from build123d import *

# Parameters (mm, degrees)
SKETCH_W    = 200
SKETCH_H    = 45
PAD_DEPTH   = 19
FILLET_R    = 5
THICKNESS_T = -1


with BuildPart() as part:
    # Sketch → Pad (new body)
    with BuildSketch(Plane.XY):
        Rectangle(SKETCH_W, SKETCH_H)
    extrude(amount=PAD_DEPTH)

    # Fillet
    fillet_edges = [part.edges().sort_by_distance(p)[0] for p in [
        (-100, -22.5, 9.5),
        (-100, 22.5, 9.5),
        (100, -22.5, 9.5),
        (100, 22.5, 9.5),
    ]]
    fillet(fillet_edges, radius=FILLET_R)

    # Thickness
    thickness_openings = [part.faces().sort_by_distance(p)[0] for p in [
        (0, 0, 19),
    ]]
    offset(amount=THICKNESS_T, openings=thickness_openings)


solid = part.part
Can you work these out from the model? Positions are in its coordinate system, mm. A direction names the side the tool comes from. Give positions to 0.01 mm unless a question says otherwise; leave off trailing zeros. Loops run counter-clockwise (first coordinate to the right, second up) from the corner with the lowest first, then second, coordinate; pieces in that order, holes last. Notation, with made-up numbers: (5, -9) - (10, -9) arc R20 ccw to (10, 6) - close; hole circle Ø4 at (84, 89). An arc over 180 degrees is marked (long way). One line per item, written item: value.
(1) On a 3-axis mill with a long thin cutter (end or side, diameter ignored), from which of +Z, -Z, +X, -X, +Y, -Y can I reach the whole of each face in a straight line? I mean faces 4 (the face through (-1, 0, 0)), 5 (the face through (-99, 0, 10)). Say none if no direction works.
Verdict:
face 4: -Z, +X, -X, +Y, -Y
face 5: +Z
(2) I'm going to push a flat-ended pin straight in: pin 1 (10 mm diameter, centred on x = -66.5, y = -7, fed in from +Z). Where does the tip first touch, or does it pass through?
Verdict:
pin 1: z = 1
(3) If we section it at C-C, the plane x = 44: List the corners of the cut face in (y, z) for me, plus the area to 3 significant figures.
Verdict:
outline: (-22.5, 0) - (22.5, 0) - (22.5, 19) - (21.5, 19) - (21.5, 1) - (-21.5, 1) - (-21.5, 19) - (-22.5, 19) - close
area: 81.0 mm^2
(4) If we mould it in two halves opening along X, with no side actions, what happens to faces 1 (the face through (-1, 21.5, 10)), 2 (the face through (-98.57, 21, 9.63)), 3 (the face through (-1, 22.5, 9))? For each: released by +X, released by -X, zero draft, split by the parting line, or undercut.
Verdict:
face 1: undercut
face 2: released by -X
face 3: zero draft
(5) If we section it at A-A, the plane y = -2.5: List the corners of the cut face in (x, z) for me, plus the area to 3 significant figures.
Verdict:
outline: (-100, 0) - (100, 0) - (100, 19) - (99, 19) - (99, 1) - (-99, 1) - (-99, 19) - (-100, 19) - close
area: 236 mm^2
(6) I need wall thicknesses on line 1 along X through (y, z) = (4, 3.75); line 2 along Y through (x, z) = (67.5, 9.25); line 3 along Z through (x, y) = (-66, 16). Which ranges of each line are inside material? Lowest first, please.
Verdict:
line 1: -100 to -99, 99 to 100
line 2: -22.5 to -21.5, 21.5 to 22.5
line 3: 0 to 1
(7) If we section it at B-B, the plane z = 15: List the corners of the cut face in (x, y) for me.
Verdict:
outline: (-100, -17.5) arc R5 ccw to (-95, -22.5) - (95, -22.5) arc R5 ccw to (100, -17.5) - (100, 17.5) arc R5 ccw to (95, 22.5) - (-95, 22.5) arc R5 ccw to (-100, 17.5) - close; hole (-99, -17.5) arc R4 ccw to (-95, -21.5) - (95, -21.5) arc R4 ccw to (99, -17.5) - (99, 17.5) arc R4 ccw to (95, 21.5) - (-95, 21.5) arc R4 ccw to (-99, 17.5) - close
